```python
from build123d import *

# Parameters (mm, degrees)
BOSS_EXTRUDE1_DEPTH = 114.3
BOSS_EXTRUDE2_START = 114.3
BOSS_EXTRUDE2_DEPTH = 1.27
SKETCH4_W           = 12.7
SKETCH4_H           = 5.08
BOSS_EXTRUDE4_DEPTH = 1.27


with BuildPart() as part:
    # Sketch1 → Boss-Extrude1 (new, symmetric)
    with BuildSketch(Plane(origin=(0, 0, 0), x_dir=(0, 0, -1), z_dir=(1, 0, 0))):
        with BuildLine():
            Line((12.7, 0), (-12.7, 0))
            Line((-12.7, 0), (-12.7, 35.56))
            ThreePointArc((-12.7, 35.56), (-11.956051224, 37.356051224), (-10.16, 38.1))
            Line((-10.16, 38.1), (-1.5875, 38.1))
            Line((-1.5875, 38.1), (-1.5875, 7.62))
            Line((-1.5875, 7.62), (-6.35, 7.62))
            Line((-6.35, 7.62), (-6.35, 2.54))
            Line((-6.35, 2.54), (6.35, 2.54))
            Line((6.35, 2.54), (6.35, 7.62))
            Line((6.35, 7.62), (1.5875, 7.62))
            Line((1.5875, 7.62), (1.5875, 38.1))
            Line((1.5875, 38.1), (10.16, 38.1))
            ThreePointArc((10.16, 38.1), (11.956051224, 37.356051224), (12.7, 35.56))
            Line((12.7, 35.56), (12.7, 0))
        make_face()
        Polygon((10.16, 35.56), (4.1275, 35.56), (4.1275, 10.16), (8.89, 10.16), (8.89, 2.54), (10.16, 2.54), align=None, mode=Mode.SUBTRACT)
        Polygon((-4.1275, 10.16), (-8.89, 10.16), (-8.89, 2.54), (-10.16, 2.54), (-10.16, 35.56), (-4.1275, 35.56), align=None, mode=Mode.SUBTRACT)
    extrude(amount=BOSS_EXTRUDE1_DEPTH, both=True)

    # Sketch2 → Boss-Extrude2 (add, symmetric)
    with BuildSketch(Plane(origin=(0, 0, 0), x_dir=(0, 0, -1), z_dir=(1, 0, 0)).offset(BOSS_EXTRUDE2_START)):
        with BuildLine():
            Line((-12.7, 0), (12.7, 0))
            Line((12.7, 0), (12.7, 35.56))
            ThreePointArc((12.7, 35.56), (11.956051224, 37.356051224), (10.16, 38.1))
            Line((10.16, 38.1), (-10.16, 38.1))
            ThreePointArc((-10.16, 38.1), (-11.956051224, 37.356051224), (-12.7, 35.56))
            Line((-12.7, 35.56), (-12.7, 0))
        make_face()
    extrude(amount=BOSS_EXTRUDE2_DEPTH, both=True)

    # Sketch4 → Boss-Extrude4 (add, symmetric)
    with BuildSketch(Plane.ZY.offset(114.3)):
        with BuildLine():
            Line((-12.7, 0), (12.7, 0))
            Line((12.7, 0), (12.7, 35.56))
            ThreePointArc((12.7, 35.56), (11.956051224, 37.356051224), (10.16, 38.1))
            Line((10.16, 38.1), (-10.16, 38.1))
            ThreePointArc((-10.16, 38.1), (-11.956051224, 37.356051224), (-12.7, 35.56))
            Line((-12.7, 35.56), (-12.7, 0))
        make_face()
        with Locations((0, 5.08)):
            Rectangle(SKETCH4_W, SKETCH4_H, mode=Mode.SUBTRACT)
    extrude(amount=BOSS_EXTRUDE4_DEPTH, both=True)


solid = part.part
```
The model under review builds one solid part; all positions refer to its coordinate system, in mm. A direction names the side the tool comes from. Coordinates: 2 decimals unless noted, no trailing zeros. Write each loop counter-clockwise with the first axis right and the second up, starting at its lowest first coordinate (ties: lowest second). Pieces come first, ordered by that corner, then holes. Notation, with made-up numbers: (41.25, -16) - (54.25, -16) arc R27 ccw to (54.25, 10) - close; hole circle Ø7 at (-28, 64). An arc over 180 degrees is marked (long way). Write item = value, one per line.
(1) For line 1 (Z direction, x = 93.5, y = 31.5); line 2 (Y direction, x = 93, z = -6.25); line 3 (Z direction, x = 41, y = 10), list the stretches that pass through material, from the lowest coordinate up. Write a range as [from, to].
Result sheet:
line_1 = [-12.7, -10.16], [-4.13, -1.59], [1.59, 4.13], [10.16, 12.7]
line_2 = [0, 2.54], [7.62, 10.16], [35.56, 38.1]
line_3 = [-12.7, -10.16], [-8.89, -1.59], [1.59, 8.89], [10.16, 12.7]
(2) Consider section C-C, the plane y = 32. Give the boundary of the cut face in (x, z), then the cut area to 3 significant figures.
Result sheet:
outline = (-115.57, -12.7) - (115.57, -12.7) - (115.57, 12.7) - (-115.57, 12.7) - close; hole (-113.03, -10.16) - (113.03, -10.16) - (113.03, -4.13) - (-113.03, -4.13) - close; hole (-113.03, -1.59) - (113.03, -1.59) - (113.03, 1.59) - (-113.03, 1.59) - close; hole (-113.03, 4.13) - (113.03, 4.13) - (113.03, 10.16) - (-113.03, 10.16) - close
area = 2,430 mm^2
(3) Machinability: for faces 4 (the face through (2, 23, 1.588)), 5 (the face through (2, 35.56, 7)), 6 (the face through (-3, 2.54, 0)), which of the approach directions +Z, -Z, +X, -X, +Y, -Y give a long, thin tool a straight path to every point of the face, cutting with its end or side? Answer none if there is none.
Result sheet:
face_4 = +Y
face_5 = none
face_6 = -X
(4) Consider section B-B, the plane x = 31.5. Give the boundary of the cut face in (y, z), then the cut area to 3 significant figures.
Result sheet:
outline = (0, -12.7) - (35.56, -12.7) arc R2.54 ccw to (38.1, -10.16) - (38.1, -1.59) - (7.62, -1.59) - (7.62, -6.35) - (2.54, -6.35) - (2.54, 6.35) - (7.62, 6.35) - (7.62, 1.59) - (38.1, 1.59) - (38.1, 10.16) arc R2.54 ccw to (35.56, 12.7) - (0, 12.7) - close; hole (2.54, -10.16) - (35.56, -10.16) - (35.56, -4.13) - (10.16, -4.13) - (10.16, -8.89) - (2.54, -8.89) - close; hole (2.54, 8.89) - (10.16, 8.89) - (10.16, 4.13) - (35.56, 4.13) - (35.56, 10.16) - (2.54, 10.16) - close
area = 478 mm^2
(5) Mouldability with a two-part tool opening along Z and no side actions: class faces 1 (the face through (2, 18, 12.7)), 2 (the face through (113.03, 17, 0)), 3 (the face through (2, 18, -12.7)) as pulls with the +Z half, pulls with the -Z half, needs draft (parallel to the pull), parting line crosses it, or undercut.
Result sheet:
face_1 = pulls with the +Z half
face_2 = undercut
face_3 = pulls with the -Z half
(6) Consider section A-A, the plane y = 5.5. Give the boundary of the cut face in (x, z).
Result sheet:
outline = (-115.57, -12.7) - (115.57, -12.7) - (115.57, 12.7) - (-115.57, 12.7) - (-115.57, 6.35) - (113.03, 6.35) - (113.03, -6.35) - (-115.57, -6.35) - close; hole (-113.03, -10.16) - (113.03, -10.16) - (113.03, -8.89) - (-113.03, -8.89) - close; hole (-113.03, 8.89) - (113.03, 8.89) - (113.03, 10.16) - (-113.03, 10.16) - close
